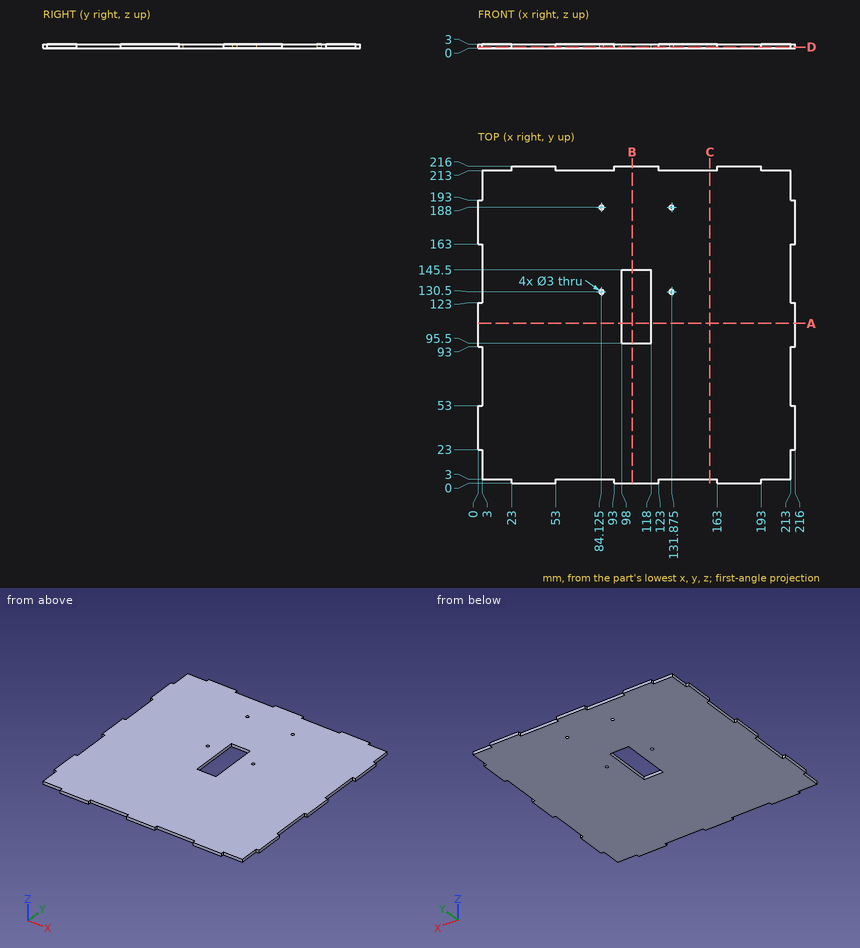
Source: three-view drawing plus pictorial views. Frame: mm from the lowest corner of the part. Round coordinates to 2 decimals unless told otherwise and drop trailing zeros. Loops run counter-clockwise (first coordinate to the right, second up) from the corner with the lowest first, then second, coordinate; pieces in that order, holes last.
Q1. Section A-A on y = 109. Return loops of the section in (x, z).
Q2. Pin query (flat end, axial travel): P1, Ø1.5, axis at y = 215, z = 1, coming from the +X side; P2, Ø0.9, axis at x = 206, z = 1, coming from the -Y side. Return the tip coordinate at first contact, or that it passes through.
Q3. Section C-C on x = 158. Return loops of the section in (y, z).
Q4. Material intervals for L1, parallel to X at y = 130.5, z = 1.9 (3 decimals); L2, parallel to X at y = 134.5, z = 2.6; L3, parallel to X at y = 121.5, z = 0.4, sorted ascending.
Q5. Section B-B on x = 105. Return loops of the section in (y, z), plus the area to 3 significant figures.
Q6. Section D-D on z = 0.95. State how many separate pieces and enclosed holes the cut face has, plus the area to 3 significant figures.
Evaluation:
1. outline: (0, 0) - (98, 0) - (98, 3) - (0, 3) - close; (118, 0) - (216, 0) - (216, 3) - (118, 3) - close
2. P1: stops at x = 193
2. P2: stops at y = 3
3. outline: (3, 0) - (213, 0) - (213, 3) - (3, 3) - close
4. L1: x = 3 to 82.625, 85.625 to 98, 118 to 130.375, 133.375 to 213
4. L2: x = 3 to 98, 118 to 213
4. L3: x = 0 to 98, 118 to 216
5. outline: (0, 0) - (95.5, 0) - (95.5, 3) - (0, 3) - close; (145.5, 0) - (216, 0) - (216, 3) - (145.5, 3) - close
5. area: 498 mm2
6. separate pieces: 1
6. enclosed holes: 5
6. area: 44,200 mm2
